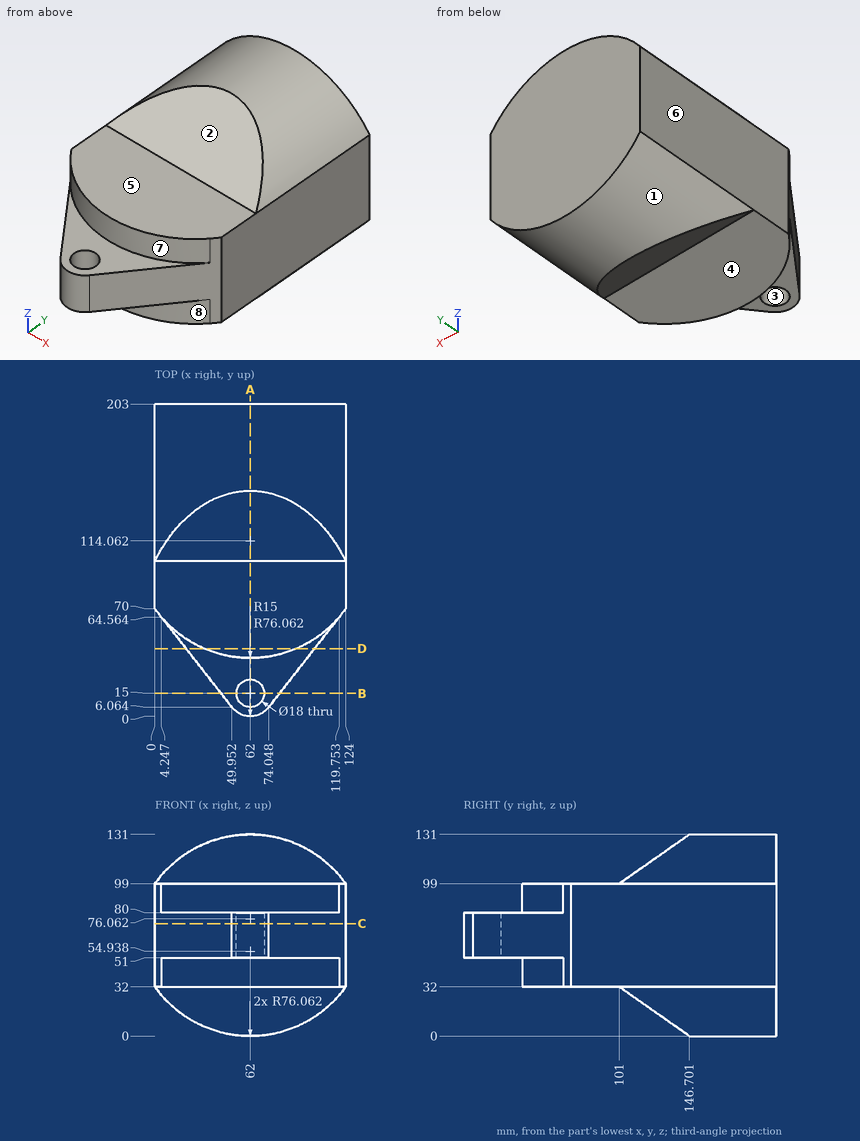
Design review of the part shown in the three views and the two pictorial views. Dimensions are in mm from the part's minimum x, y and z. A direction names the side the tool comes from. Coordinates: 2 decimals unless noted, no trailing zeros. Write each loop counter-clockwise with the first axis right and the second up, starting at its lowest first coordinate (ties: lowest second). Pieces come first, ordered by that corner, then holes.
1) To check wall thickness, follow probe 1 along Z at (x, y) = (70.5, 60.5); probe 2 along Z at (x, y) = (61.5, 191); probe 3 along Y at (x, z) = (37, 124) (1 decimal). State the ranges of each line that lie inside material, in increasing order.
2) We need section C-C on z = 73. State the section outline as (x, y) points (1 decimal), then the cut area to 3 significant figures.
3) We need section B-B on y = 15. State the section outline as (x, z) points.
4) The part is to be moulded in two halves that separate along X. For the marked faces 1, 2 and 3, say which applies: pulls with the +X half, pulls with the -X half, needs draft (parallel to the pull), parting line crosses it, or undercut.
5) We need section A-A on x = 62. State the section outline as (y, z) points, then the cut area to 3 significant figures.
6) Machinability: for the marked faces 4, 5, 6, 7 and 8, which of the approach directions +Z, -Z, +X, -X, +Y, -Y give a long, thin tool a straight path to every point of the face, cutting with its end or side? Answer none if there is none.
7) We need section D-D on y = 44. State the section outline as (x, z) points, then the cut area to 3 significant figures.
8) Clearance check with flat-ended pins moving along their axes: pin 1 Ø19 at (x, y) = (33.5, 75) entering from +Z; pin 2 Ø4 at (x, y) = (104.5, 141) entering from +Z; pin 3 Ø8 at (x, z) = (50.5, 15.5) entering from -Y; pin 4 Ø16 at (x, y) = (62, 15) entering from +Z. State where each tip first meets the part, or that it passes through.
Answer list:
1. probe 1: z = 32 to 99
1. probe 2: z = 0 to 131
1. probe 3: y = 136.7 to 203
2. outline: (0, 70) - (50, 6.1) arc R15 ccw to (74, 6.1) - (124, 70) - (124, 203) - (0, 203) - close; hole circle Ø18 at (62, 15)
2. area: 21,100 mm2
3. outline: (42.97, 51) - (53, 51) - (53, 80) - (42.97, 80) - close; (71, 51) - (81.03, 51) - (81.03, 80) - (71, 80) - close
4. face 1: parting line crosses it
4. face 2: needs draft
4. face 3: undercut
5. outline: (0, 51) - (6, 51) - (6, 80) - (0, 80) - close; (24, 51) - (38, 51) - (38, 32) - (101, 32) - (146.7, 0) - (203, 0) - (203, 131) - (146.7, 131) - (101, 99) - (38, 99) - (38, 80) - (24, 80) - close
5. area: 16,700 mm2
6. face 4: -Z, +X, -X, -Y
6. face 5: +Z, +X, -X, -Y
6. face 6: +Z, -Z, -X, +Y, -Y
6. face 7: +Z, -Y
6. face 8: -Z, -Y
7. outline: (20.31, 51) - (32.39, 51) - (32.39, 32) - (91.61, 32) - (91.61, 51) - (103.69, 51) - (103.69, 80) - (91.61, 80) - (91.61, 99) - (32.39, 99) - (32.39, 80) - (20.31, 80) - close
7. area: 4,670 mm2
8. pin 1: stops at z = 99
8. pin 2: stops at z = 119.32
8. pin 3: stops at y = 118.85
8. pin 4: passes through
